from build123d import *

# Parameters (mm, degrees)
CYLINDER063_R     = 1.5
CYLINDER063_DEPTH = 11
CYLINDER062_R     = 13.5
CYLINDER062_DEPTH = 19.5


with BuildPart() as servo_pot_shaft:
    # Cylinder063 → Cylinder063 (new body)
    with BuildSketch(Plane.XY.offset(19.5)):
        Circle(CYLINDER063_R)
    extrude(amount=CYLINDER063_DEPTH)


with BuildPart() as servo_pot:
    # Cylinder062 → Cylinder062 (new body)
    with BuildSketch(Plane.XY):
        Circle(CYLINDER062_R)
    extrude(amount=CYLINDER062_DEPTH)

    # Fusion027: union servo-pot-shaft
    add(servo_pot_shaft.part)


with BuildPart() as servo_pot_1:
    # Fusion027 placement: moved
    add(servo_pot.part.moved(Location((0, 0, 16.7))))


solid = servo_pot_1.part
Can you work these out from the model? Positions are in its coordinate system, mm. A direction names the side the tool comes from. Coordinates: 2 decimals unless noted, no trailing zeros. Write each loop counter-clockwise with the first axis right and the second up, starting at its lowest first coordinate (ties: lowest second). Pieces come first, ordered by that corner, then holes. Notation, with made-up numbers: (64, 7) -> (72, 7) arc R23 cw to (72, 18) -> close; hole circle Ø1 at (13, 15.25). An arc over 180 degrees is marked (long way). Write item = value, one per line.
(1) Imagine slicing it at D-D (z = 37.5). Please give me the cut outline in (x, y), and give its area (3 significant figures).
Verdict:
outline = circle Ø3 at (0, 0)
area = 7.07 mm^2
(2) Imagine slicing it at C-C (z = 33). Please give me the cut outline in (x, y).
Verdict:
outline = circle Ø27 at (0, 0)
(3) If I drill on probe 1 along Z at (x, y) = (3.5, -7.5); probe 2 along X at (y, z) = (-8.25, 35); probe 3 along Y at (x, z) = (-9.75, 29.5), over which ranges is the centre line in solid material (lowest first)?
Verdict:
probe_1 = 16.7 to 36.2
probe_2 = -10.69 to 10.69
probe_3 = -9.34 to 9.34
(4) Thinking about a two-plate mould opening in Y: for faces 3 (the face through (0, 0, 47.2)), 4 (the face through (-2.93, -13.18, 26.31)), which applies, +Y half, -Y half, draft (parallel to the pull), parting line (faces both ways), or undercut?
Verdict:
face_3 = draft
face_4 = parting line
(5) On a 3-axis mill with a long thin cutter (end or side, diameter ignored), from which of +Z, -Z, +X, -X, +Y, -Y can I reach the whole of each face in a straight line? I mean faces 1 (the face through (0, 0, 16.7)), 2 (the face through (-1.5, 0.07, 41.62)). Say none if no direction works.
Verdict:
face_1 = -Z, +X, -X, +Y, -Y
face_2 = +Z
(6) For pin 1 (12 mm diameter, centred on y = 9, z = 20, fed in from -X); pin 2 (12 mm diameter, centred on x = -7, z = 26.5, fed in from +Y); pin 3 (3 mm diameter, centred on x = -3, y = 4.5, fed in from +Z), each with a flat end and sliding along its axis, tell me the tip position at first contact or that it passes through.
Verdict:
pin_1 = -13.16
pin_2 = 13.46
pin_3 = 36.2
(7) Imagine slicing it at A-A (y = 0). Please give me the cut outline in (x, z).
Verdict:
outline = (-13.5, 16.7) -> (13.5, 16.7) -> (13.5, 36.2) -> (1.5, 36.2) -> (1.5, 47.2) -> (-1.5, 47.2) -> (-1.5, 36.2) -> (-13.5, 36.2) -> close
